from build123d import *

# Parameters (mm, degrees)
BASE_FLANGE1_DEPTH                        = 1219.2
F_10_0_1935_DIAMETER_HOLE1_D              = 4.9149
HOLE_FOR_1_4_SELF_CLINCHING_NUTS_S_SS_C_D = 8.7376
SKETCH15_W                                = 38.1
SKETCH15_H                                = 22.86
CUT_EXTRUDE4_DEPTH                        = 5.76326
SKETCH16_W                                = 107.95
SKETCH16_H                                = 5.76326
SKETCH16_W_2                              = 171.45
CUT_EXTRUDE5_DEPTH                        = 1222.511012488
HOLE_FOR_1_4_SELF_CLINCHING_NUTS_S_2_D    = 8.7376
CUT_EXTRUDE7_REACH                        = 1224.598
SKETCH27_W                                = 63.5
SKETCH27_H                                = 26.035
SKETCH28_W                                = 60.325
SKETCH28_H                                = 58.95848
CUT_EXTRUDE8_DEPTH                        = 1223.597502808
SKETCH32_W                                = 38.1
SKETCH32_H                                = 5.76326
CUT_EXTRUDE9_DEPTH                        = 1055.864621408
SKETCH30_W                                = 1098.55
SKETCH30_H                                = 4.17576
BOSS_EXTRUDE1_DEPTH                       = 2.58826
FILLET1_R                                 = 2.54


# Read off the part's stored shape, not the designer's step: Base-Flange1
with BuildPart() as part:
    # Base-Flange1 outline → Base-Flange1 (new body)
    with BuildSketch(Plane(origin=(0, 0, 0), x_dir=(0, 0, -1), z_dir=(1, 0, 0))):
        with BuildLine():
            Line((61.49848, -47.625), (61.49848, -64.72174))
            Line((61.49848, -64.72174), (64.08674, -64.72174))
            Line((64.08674, -64.72174), (64.08674, -47.625))
            ThreePointArc((64.08674, -47.625), (62.398720228, -43.549759772), (58.32348, -41.86174))
            Line((58.32348, -41.86174), (41.275, -41.86174))
            ThreePointArc((41.275, -41.86174), (39.02993597, -40.93180403), (38.1, -38.68674))
            Line((38.1, -38.68674), (38.1, -5.76326))
            ThreePointArc((38.1, -5.76326), (36.411980228, -1.688019772), (32.33674, 0))
            Line((32.33674, 0), (0, 0))
            Line((0, 0), (0, -2.58826))
            Line((0, -2.58826), (32.33674, -2.58826))
            ThreePointArc((32.33674, -2.58826), (34.58180403, -3.51819597), (35.51174, -5.76326))
            Line((35.51174, -5.76326), (35.51174, -38.68674))
            ThreePointArc((35.51174, -38.68674), (37.199759772, -42.761980228), (41.275, -44.45))
            Line((41.275, -44.45), (58.32348, -44.45))
            ThreePointArc((58.32348, -44.45), (60.56854403, -45.37993597), (61.49848, -47.625))
        make_face()
    extrude(amount=BASE_FLANGE1_DEPTH)

    # #10 (0.1935) Diameter Hole1 (through all)
    with Locations(Plane(origin=(0, 0, -38.1), x_dir=(-1, 0, 0), z_dir=(0, 0, -1))):
        with Locations((-146.05, -12.7), (-609.6, -12.7), (-609.6, -31.75), (-1073.15, -12.7), (-1073.15, -31.75), (-146.05, -31.75)):
            Hole(F_10_0_1935_DIAMETER_HOLE1_D / 2)

    # Hole for 1_4 Self-clinching Nuts _S_SS_C (through all)
    with Locations(Plane(origin=(0, -2.58826, 0), x_dir=(-1, 0, 0), z_dir=(0, -1, 0))):
        with Locations((-304.8, 13.28674), (-914.4, 13.28674)):
            Hole(HOLE_FOR_1_4_SELF_CLINCHING_NUTS_S_SS_C_D / 2)

    # Sketch15 → Cut-Extrude4 (cut)
    with BuildSketch(Plane(origin=(0, 0, -64.08674), x_dir=(-1, 0, 0), z_dir=(0, 0, -1))):
        with Locations((-1200.15, -53.29174)):
            Rectangle(SKETCH15_W, SKETCH15_H)
        with Locations((-19.05, -53.29174)):
            Rectangle(SKETCH15_W, SKETCH15_H)
    extrude(amount=-CUT_EXTRUDE4_DEPTH, mode=Mode.SUBTRACT)

    # Sketch16 → Cut-Extrude5 (cut, through all)
    with BuildSketch(Plane(origin=(0, 0, -38.1), x_dir=(-1, 0, 0), z_dir=(0, 0, -1))):
        with Locations((-1165.225, -2.88163)):
            Rectangle(SKETCH16_W, SKETCH16_H)
        with Locations((-609.6, -2.88163)):
            Rectangle(SKETCH16_W_2, SKETCH16_H)
        with Locations((-53.975, -2.88163)):
            Rectangle(SKETCH16_W, SKETCH16_H)
    extrude(amount=-CUT_EXTRUDE5_DEPTH, mode=Mode.SUBTRACT)

    # Hole for 1_4 Self-clinching Nuts _S_ 2 (through all)
    with Locations(Plane(origin=(0, 0, -64.08674), x_dir=(-1, 0, 0), z_dir=(0, 0, -1))):
        with Locations((-1143, -56.78424), (-863.6, -56.78424), (-355.6, -56.78424), (-76.2, -56.78424)):
            Hole(HOLE_FOR_1_4_SELF_CLINCHING_NUTS_S_2_D / 2)

    # Cut-Extrude7: up to this face of the body (flat: up to its plane)
    cut_extrude7_end = Plane(part.part.faces().sort_by_distance((609.6, -22.225, -35.51174))[0])
    # Sketch27 → Cut-Extrude7 (cut, up to the picked face)
    with BuildSketch(Plane.XY.offset(-64.08674), mode=Mode.PRIVATE) as cut_extrude7_sk1:
        with Locations((146.05, -51.70424)):
            Rectangle(SKETCH27_W, SKETCH27_H)
    cut_extrude7_tool1 = split(extrude(cut_extrude7_sk1.sketch, amount=CUT_EXTRUDE7_REACH, mode=Mode.PRIVATE), bisect_by=cut_extrude7_end, keep=Keep.BOTH, mode=Mode.PRIVATE)
    # Sketch27 → Cut-Extrude7 (cut, up to the picked face)
    with BuildSketch(Plane.XY.offset(-64.08674), mode=Mode.PRIVATE) as cut_extrude7_sk2:
        with Locations((1073.15, -51.70424)):
            Rectangle(SKETCH27_W, SKETCH27_H)
    cut_extrude7_tool2 = split(extrude(cut_extrude7_sk2.sketch, amount=CUT_EXTRUDE7_REACH, mode=Mode.PRIVATE), bisect_by=cut_extrude7_end, keep=Keep.BOTH, mode=Mode.PRIVATE)
    # Sketch27 → Cut-Extrude7 (cut, up to the picked face)
    with BuildSketch(Plane.XY.offset(-64.08674), mode=Mode.PRIVATE) as cut_extrude7_sk3:
        with Locations((609.6, -51.70424)):
            Rectangle(SKETCH27_W, SKETCH27_H)
    cut_extrude7_tool3 = split(extrude(cut_extrude7_sk3.sketch, amount=CUT_EXTRUDE7_REACH, mode=Mode.PRIVATE), bisect_by=cut_extrude7_end, keep=Keep.BOTH, mode=Mode.PRIVATE)
    add(cut_extrude7_tool1.solids().sort_by(Axis((146.05, -51.70424, -64.08674), (0, 0, 1)))[0], mode=Mode.SUBTRACT)
    add(cut_extrude7_tool2.solids().sort_by(Axis((1073.15, -51.70424, -64.08674), (0, 0, 1)))[0], mode=Mode.SUBTRACT)
    add(cut_extrude7_tool3.solids().sort_by(Axis((609.6, -51.70424, -64.08674), (0, 0, 1)))[0], mode=Mode.SUBTRACT)

    # Sketch28 → Cut-Extrude8 (cut, through all)
    with BuildSketch(Plane(origin=(0, 0, -64.08674), x_dir=(-1, 0, 0), z_dir=(0, 0, -1))):
        with Locations((-1189.0375, -35.2425)):
            Rectangle(SKETCH28_W, SKETCH28_H)
        with Locations((-30.1625, -35.2425)):
            Rectangle(SKETCH28_W, SKETCH28_H)
    extrude(amount=-CUT_EXTRUDE8_DEPTH, mode=Mode.SUBTRACT)

    # Sketch32 → Cut-Extrude9 (cut, through all)
    with BuildSketch(Plane(origin=(1111.25, 0, 0), x_dir=(0, 0, -1), z_dir=(1, 0, 0))):
        with Locations((19.05, -2.88163)):
            Rectangle(SKETCH32_W, SKETCH32_H)
    extrude(amount=-CUT_EXTRUDE9_DEPTH, mode=Mode.SUBTRACT)

    # Sketch30 → Boss-Extrude1 (add)
    with BuildSketch(Plane(origin=(0, 0, -38.1), x_dir=(-1, 0, 0), z_dir=(0, 0, -1))):
        with Locations((-609.6, -3.67538)):
            Rectangle(SKETCH30_W, SKETCH30_H)
    extrude(amount=-BOSS_EXTRUDE1_DEPTH)

    # Fillet1
    fillet1_edges = [part.edges().sort_by_distance(p)[0] for p in [
        (1041.4, -64.72174, -62.79261),
        (1158.875, -1.5875, -36.80587),
        (60.325, -1.5875, -36.80587),
        (177.8, -64.72174, -62.79261),
        (60.325, -64.72174, -62.79261),
        (641.35, -64.72174, -62.79261),
        (1104.9, -64.72174, -62.79261),
        (1158.875, -64.72174, -62.79261),
        (114.3, -64.72174, -62.79261),
        (577.85, -64.72174, -62.79261),
    ]]
    fillet(fillet1_edges, radius=FILLET1_R)


solid = part.part
Can you work these out from the model? Positions are in its coordinate system, mm. A direction names the side the tool comes from. Give positions to 0.01 mm unless a question says otherwise; leave off trailing zeros. Loops run counter-clockwise (first coordinate to the right, second up) from the corner with the lowest first, then second, coordinate; pieces in that order, holes last. Notation, with made-up numbers: M 82,39.5 L 102,39.5 A33 cw 102,67.5 Z; hole C -35.5,72.25 d3. An arc over 180 degrees is marked long. One line per item, written item: value.
1) On a 3-axis mill with a long thin cutter (end or side, diameter ignored), from which of +Z, -Z, +X, -X, +Y, -Y can I reach the whole of each face in a straight line? I mean faces 3 (the face through (87, -41.862, -50)), 4 (the face through (839, -44.45, -50)), 5 (the face through (617, -20, -35.512)). Say none if no direction works.
Geometry check:
face 3: -Z, +X, -X, +Y
face 4: +Z, +X, -X, -Y
face 5: +Z, +X, -X, +Y, -Y
2) Please list where these lines run through material, in increasing order: line 1 (Y direction, x = 146.05, z = -37.1); line 2 (Y direction, x = 76.2, z = -63.25); line 3 (X direction, y = -11.5, z = -38) (3 decimals).
Geometry check:
line 1: y = -38.69 to -34.21, -29.29 to -15.16, -10.24 to -1.59
line 2: y = -64.72 to -61.15, -52.42 to -44.63
line 3: x = 60.325 to 143.905, 148.195 to 607.455, 611.745 to 1071.005, 1075.295 to 1158.875
3) Imagine slicing it at A-A on z = -48.25. Write out the boundary of the cut face in (x, y) (3 decimals).
Geometry check:
outline: M 60.325,-44.45 L 114.3,-44.45 L 114.3,-41.862 L 60.325,-41.862 Z; M 177.8,-44.45 L 577.85,-44.45 L 577.85,-41.862 L 177.8,-41.862 Z; M 641.35,-44.45 L 1041.4,-44.45 L 1041.4,-41.862 L 641.35,-41.862 Z; M 1104.9,-44.45 L 1158.875,-44.45 L 1158.875,-41.862 L 1104.9,-41.862 Z
4) Thinking about a two-plate mould opening in X: for faces 1 (the face through (617, -20, -38.1)), 2 (the face through (577.85, -44, -55)), which applies, +X half, -X half, draft (parallel to the pull), parting line (faces both ways), or undercut?
Geometry check:
face 1: draft
face 2: undercut
5) I'm going to push flat-ended pins straight in: pin 1 (1 mm diameter, centred on x = 747.5, y = -12, fed in from -Z); pin 2 (8.5 mm diameter, centred on x = 95.5, y = -55, fed in from +Z); pin 3 (5 mm diameter, centred on x = 98.5, z = -49.5, fed in from +Y); pin 4 (8 mm diameter, centred on y = -42, z = -60.5, fed in from -X) (3 decimals). Where does each tip first touch, or does it pass through?
Geometry check:
pin 1: stops at z = -38.1
pin 2: stops at z = -61.5
pin 3: stops at y = -41.86
pin 4: stops at x = 60.325
